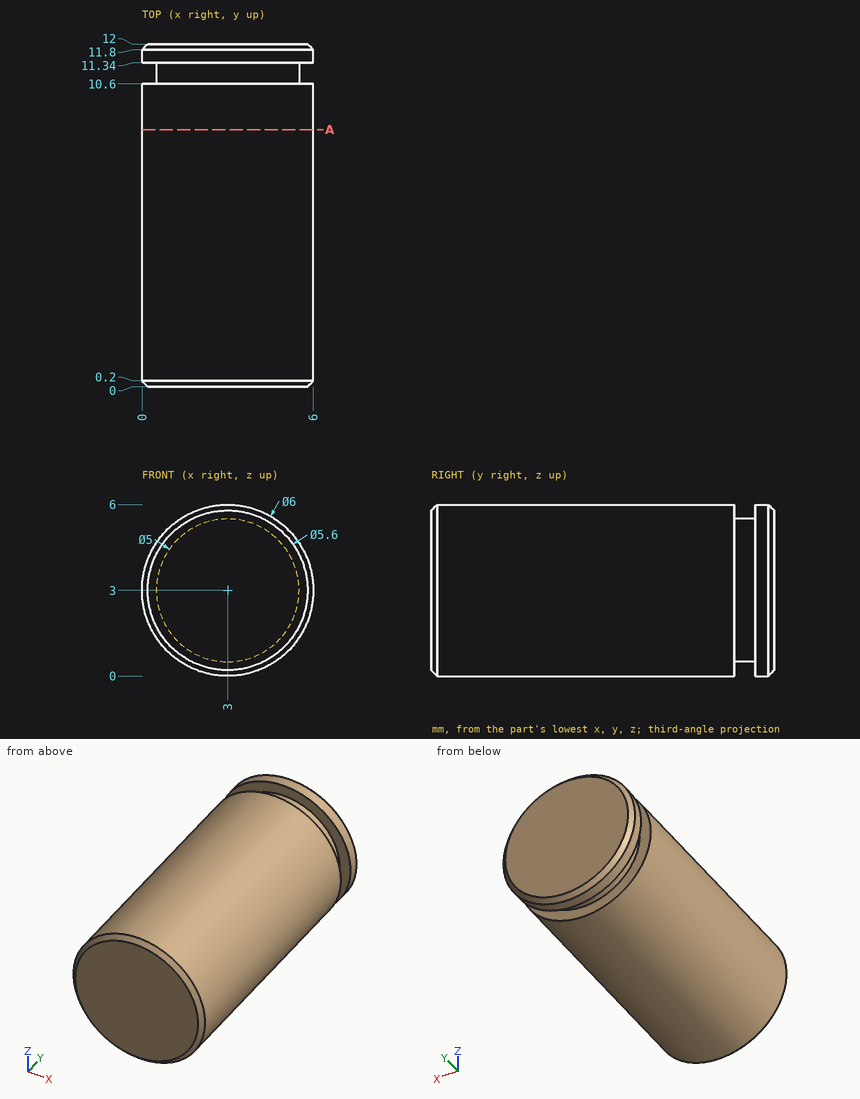
Study the drawing (mm; zero at the part's minimum x, y, z) and answer. Give positions to 0.01 mm unless a question says otherwise; leave off trailing zeros. Write each loop counter-clockwise with the first axis right and the second up, starting at its lowest first coordinate (ties: lowest second). Pieces come first, ordered by that corner, then holes. Notation, with made-up numbers: (-25.75, 77) - (13.25, 77) arc R21 ccw to (13.25, 89) - close; hole circle Ø9 at (-26.5, 78.25). An arc over 180 degrees is marked (long way). One line per question, with ' | ' between items. Start each with the question number.
1. Straight lines are drawn through the part: line 1 (Y direction, x = 4.5, z = 5.05); line 2 (Y direction, x = 5.45, z = 4.5); line 3 (X direction, y = 3.5, z = 0.6). For each, find the intervals that lie inside material, in ascending order.
2. Given P1, Ø1, axis at y = 9.5, z = 1.5, coming from the -X side; P2, Ø1, axis at y = 5.5, z = 2, coming from the -X side, each flat-ended and moving along its own axis, determine where each tip first touches the part or whether it passes through.
3. Section A-A, the plane y = 9 is taken. Determine the outline of the cut face in (x, z).
Result:
1) line 1: y = 0 to 10.6, 11.34 to 12 | line 2: y = 0.07 to 10.6, 11.34 to 11.93 | line 3: x = 1.2 to 4.8
2) P1: stops at x = 0.17 | P2: stops at x = 0.04
3) outline: circle Ø6 at (3, 3)
